Input: part model. Units: mm. Frame: model coordinates. A direction names the side the tool comes from. Give positions to 0.01 mm unless a question says otherwise; leave off trailing zeros. Loops run counter-clockwise (first coordinate to the right, second up) from the corner with the lowest first, then second, coordinate; pieces in that order, holes last. Notation, with made-up numbers: (13.25, 82.25) - (44.25, 82.25) arc R18 cw to (44.25, 100.25) - close; hole circle Ø10 at (54, 87). An arc over 180 degrees is marked (long way). Answer as a JSON object with one key per item and string values. Group by question number.
(1) Section query D-D (z = -115). Return loops of the section in (x, y), plus the area to 3 significant figures.
(2) Section query C-C (z = -93). Return loops of the section in (x, y).
(3) Pin query (flat end, axial travel): P1, Ø3.5, axis at y = -58, z = -101.5, coming from the +X side (3 decimals); P2, Ø3, axis at x = 3.5, z = -89, coming from the +Y side; P3, Ø20.5, axis at y = 61, z = -102.5, coming from the +X side; P4, Ø4, axis at x = 7, z = -100, coming from the -Y side. Return the tip coordinate at first contact, or that it passes through.
(4) Material intervals for L1, parallel to Z at x = 4.35, y = 58.5; L2, parallel to Y at x = 4.75, z = -120.5; L3, parallel to X at y = -64, z = -117, sorted ascending.
(5) Section query A-A (y = 58.5). Return loops of the section in (x, z).
(6) Section query B-B (x = 7.75). Return loops of the section in (y, z).
(7) Mould query, pull axis Y, two halves, no side actions, for faces 1 (the flat face through (6.41, 88.13, -91.3)), 2 (the flat face through (13, 0, -110)), 3 (the flat face through (4, -63, -106)), 4 (the cylindrical face through (6.409, -99.676, -105.094)). Classes: +Y half, -Y half, draft (parallel to the pull), parting line (faces both ways), or undercut.
(8) Access query for faces 5 (the cylindrical face through (6.409, 99.694, -105.141)), 6 (the flat face through (6, 63, -103)), 7 (the flat face through (4, 63, -106)). Directions: +Z, -Z, +X, -X, +Y, -Y. A direction counts if a zero-diameter tool reaches every point of the face in a straight line with its end or side. Return the directions, or none.
```python
from build123d import *

# Parameters (mm, degrees)
F0_R     = 6.2
F0_R_2   = 4.1
F1_DEPTH = 6
F2_DEPTH = 4
F3_DEPTH = 13


with BuildPart() as f1:
    # F0 (on Right) → F1 (new body)
    with BuildSketch(Plane.YZ):
        with Locations((58.5, -101.3249722428)):
            Circle(F0_R)
        with Locations((58.5, -101.3249722428)):
            Circle(F0_R_2, mode=Mode.SUBTRACT)
    extrude(amount=F1_DEPTH)

    # F0 (on Right) → F2, piece 2 (join)
    with BuildSketch(Plane.YZ):
        with BuildLine():
            ThreePointArc((79.5, -101.3249722428), (75.7871035755, -89.4020510416), (65.9613285744, -81.6951842687))
            ThreePointArc((65.9613285744, -81.6951842687), (52.5, -90.9326673974), (37.7694406564, -97.9717783471))
            ThreePointArc((37.7694406564, -97.9717783471), (56.8179991402, -122.2575036976), (79.5, -101.3249722428))
        make_face()
        with Locations((58.5, -101.3249722428)):
            Circle(F0_R, mode=Mode.SUBTRACT)
    extrude(amount=F2_DEPTH)



with BuildPart() as f1b:
    # F0 (on Right) → F1, piece 2 (new body)
    with BuildSketch(Plane.YZ):
        with Locations((-58.5, -101.3249722428)):
            Circle(F0_R)
        with Locations((-58.5, -101.3249722428)):
            Circle(F0_R_2, mode=Mode.SUBTRACT)
    extrude(amount=F1_DEPTH)

    # F0 (on Right) → F2 (join)
    with BuildSketch(Plane.YZ):
        with BuildLine():
            ThreePointArc((-37.7694406564, -97.9717783471), (-52.5, -90.9326673974), (-65.9613285744, -81.6951842687))
            ThreePointArc((-65.9613285744, -81.6951842687), (-70.4229212012, -118.6120758183), (-37.5, -101.3249722428))
            ThreePointArc((-37.5, -101.3249722428), (-37.5674685452, -99.642971383), (-37.7694406564, -97.9717783471))
        make_face()
        with Locations((-58.5, -101.3249722428)):
            Circle(F0_R, mode=Mode.SUBTRACT)
    extrude(amount=F2_DEPTH)


with BuildPart() as f1_1:
    add(f1.part)

    add(f1b.part)  # F3 merges F1b
    # F0 (on Right) → F3 (join)
    with BuildSketch(Plane.YZ):
        with BuildLine():
            ThreePointArc((-37.5, -101.3249722428), (-70.4229212012, -118.6120758183), (-65.9613285744, -81.6951842687))
            ThreePointArc((-65.9613285744, -81.6951842687), (-68.0346725838, -79.9767674166), (-70.0632666757, -78.2057457143))
            ThreePointArc((-70.0632666757, -78.2057457143), (-73.7153806196, -76.9398097428), (-77.1787849633, -78.6560150029))
            Line((-77.1787849633, -78.6560150029), (-98.7791722555, -103.5907206196))
            ThreePointArc((-98.7791722555, -103.5907206196), (-99.6848618591, -105.1175171847), (-100, -106.8645344603))
            Line((-100, -106.8645344603), (-100, -125))
            Line((-100, -125), (0, -125))
            Line((0, -125), (100, -125))
            Line((100, -125), (100, -106.8645344603))
            ThreePointArc((100, -106.8645344603), (99.6848618591, -105.1175171847), (98.7791722555, -103.5907206196))
            Line((98.7791722555, -103.5907206196), (77.1787849633, -78.6560150029))
            ThreePointArc((77.1787849633, -78.6560150029), (73.7153806196, -76.9398097428), (70.0632666757, -78.2057457143))
            ThreePointArc((70.0632666757, -78.2057457143), (68.0346725838, -79.9767674166), (65.9613285744, -81.6951842687))
            ThreePointArc((65.9613285744, -81.6951842687), (75.7871035755, -89.4020510416), (79.5, -101.3249722428))
            ThreePointArc((79.5, -101.3249722428), (56.8179991402, -122.2575036976), (37.7694406564, -97.9717783471))
            ThreePointArc((37.7694406564, -97.9717783471), (19.2088947307, -103.2279921495), (0, -105))
            ThreePointArc((0, -105), (-19.2088947307, -103.2279921495), (-37.7694406564, -97.9717783471))
            ThreePointArc((-37.7694406564, -97.9717783471), (-37.5674685452, -99.642971383), (-37.5, -101.3249722428))
        make_face()
        with Locations((0, -115)):
            Circle(F0_R_2, mode=Mode.SUBTRACT)
    extrude(amount=F3_DEPTH)


solid = f1_1.part
```
Recorded:
{
 "1": {"outline": "(0, -100) - (13, -100) - (13, -74.44) - (4, -74.44) - (4, -42.56) - (13, -42.56) - (13, -4.1) - (0, -4.1) - close; (0, 4.1) - (13, 4.1) - (13, 42.56) - (4, 42.56) - (4, 74.44) - (13, 74.44) - (13, 100) - (0, 100) - close", "area": "1,920 mm^2"},
 "2": {"outline": "(0, -89.6) - (13, -89.6) - (13, -77.78) - (4, -77.78) - (4, -48.74) - (0, -48.74) - close; (0, 48.74) - (4, 48.74) - (4, 77.78) - (13, 77.78) - (13, 89.6) - (0, 89.6) - close"},
 "3": {"P1": "passes through", "P2": "stops at y = 87.44", "P3": "stops at x = 6", "P4": "stops at y = -97.4"},
 "4": {"L1": "z = -125 to -122.32, -107.52 to -105.42, -97.22 to -95.12", "L2": "y = -100 to -67.06, -49.94 to 49.94, 67.06 to 100", "L3": "x = 0 to 4"},
 "5": {"outline": "(0, -125) - (13, -125) - (13, -122.32) - (4, -122.32) - (4, -107.52) - (6, -107.52) - (6, -105.42) - (0, -105.42) - close; (0, -97.22) - (6, -97.22) - (6, -95.12) - (4, -95.12) - (4, -87.19) - (0, -87.19) - close"},
 "6": {"outline": "(-100, -125) - (100, -125) - (100, -106.86) arc R5 ccw to (98.78, -103.59) - (77.18, -78.66) arc R5 ccw to (70.06, -78.21) arc R105 cw to (65.96, -81.7) arc R21 cw (long way) to (37.77, -97.97) arc R105 cw to (-37.77, -97.97) arc R21 cw (long way) to (-65.96, -81.7) arc R105 cw to (-70.06, -78.21) arc R5 ccw to (-77.18, -78.66) - (-98.78, -103.59) arc R5 ccw to (-100, -106.86) - close; hole circle Ø8.2 at (0, -115)"},
 "7": {"face 1": "+Y half", "face 2": "draft", "face 3": "undercut", "face 4": "-Y half"},
 "8": {"face 5": "+Z, +X, -X, +Y", "face 6": "+Z, +X", "face 7": "+X"}
}
